Can you work these out from the model? Positions are in its coordinate system, mm. A direction names the side the tool comes from. Round coordinates to 2 decimals unless told otherwise and drop trailing zeros. Loops run counter-clockwise (first coordinate to the right, second up) from the corner with the lowest first, then second, coordinate; pieces in that order, holes last. Notation, with made-up numbers: (47.5, -33.75) - (61.5, -33.75) arc R14 cw to (61.5, -20.75) - close; hole circle Ø5 at (-22.75, -29.75). An arc over 180 degrees is marked (long way). Answer as CSV lines item,"result".
Autodesk Inventor part; units mm, degrees
ref_plane "YZ Plane" through (0, 0, 0) normal (1, 0, 0) x (0, 1, 0)
ref_plane "XZ Plane" through (0, 0, 0) normal (0, 1, 0) x (-1, 0, 0)
ref_plane "XY Plane" through (0, 0, 0) normal (0, 0, 1) x (1, 0, 0)
sketch "Sketch1" plane through (0, 0, 0) normal (0, 0, 1) x (1, 0, 0)
  line L0 (4, 0) -> (76, 0)
  line L1 (80, 4) -> (80, 87.5)
  line L2 (76, 91.5) -> (4, 91.5)
  line L3 (0, 87.5) -> (0, 4)
  line L4 (0, 4) -> (4, 0)
  line L5 (76, 0) -> (80, 4)
  line L6 (80, 87.5) -> (76, 91.5)
  line L7 (4, 91.5) -> (0, 87.5)
  line L8 (16.5, 75) -> (63.5, 75)
  line L9 (64.5, 74) -> (64.5, 65)
  line L10 (63.5, 64) -> (16.5, 64)
  line L11 (15.5, 65) -> (15.5, 74)
  arc A0 (15.5, 65) -> (16.5, 64) centre (16.5, 65) ccw
  arc A1 (16.5, 75) -> (15.5, 74) centre (16.5, 74) ccw
  arc A2 (64.5, 74) -> (63.5, 75) centre (63.5, 74) ccw
  arc A3 (63.5, 64) -> (64.5, 65) centre (63.5, 65) ccw
  line L12 (28.5, 21) -> (51.5, 21)
  line L13 (52.5, 20) -> (52.5, 11)
  line L14 (51.5, 10) -> (28.5, 10)
  line L15 (27.5, 11) -> (27.5, 20)
  arc A4 (27.5, 11) -> (28.5, 10) centre (28.5, 11) ccw
  arc A5 (28.5, 21) -> (27.5, 20) centre (28.5, 20) ccw
  arc A6 (52.5, 20) -> (51.5, 21) centre (51.5, 20) ccw
  arc A7 (51.5, 10) -> (52.5, 11) centre (51.5, 11) ccw
  line L16 (15.5, 69.5) -> (64.5, 69.5) construction
  line L17 (27.5, 15.5) -> (52.5, 15.5) construction
  circle A8 centre (40, 5) radius 2.25
  circle A9 centre (10, 78.5) radius 2.25
  circle A10 centre (6, 23.25) radius 2.25
  circle A11 centre (74, 23.25) radius 2.25
  circle A12 centre (70, 78.5) radius 2.25
  point P0 (0, 0)
  point P1 (40, 64)
  point P2 (40, 21)
  point P3 (40, 75)
  point P4 (40, 91.5)
  point P5 (0, 45.75)
  point P6 (80, 45.75)
  dimension "d0" = 45
  dimension "d1" = 4
  dimension "d2" = 1
  dimension "d3" = 11
  dimension "d4" = 49
  dimension "d5" = 1
  dimension "d6" = 11
  dimension "d7" = 25
  dimension "d9" = 10
  dimension "d10" = 16.5
  dimension "d11" = 4.5
  dimension "d12" = 4.5
  dimension "d13" = 5
  dimension "d15" = 4.5
  dimension "d16" = 4.5
  dimension "d19" = 54
  dimension "d22" = 80
  dimension "d23" = 6
  dimension "d24" = 6
  dimension "d25" = 23.25
  dimension "d26" = 4.5
  dimension "d27" = 10
  dimension "d28" = 10
  dimension "d54" = 3.5
extrude "Extrusion2" add sketch "Sketch1" along normal blind 6
sketch "Sketch2" plane through (0, 0, 6) normal (0, 0, 1) x (1, 0, 0)
  line L0 (4, 0) -> (76, 0)
  circle A0 centre (20, 35) radius 2.25
  circle A1 centre (60, 35) radius 2.25
  line L1 (20, 35) -> (60, 35) construction
  point P0 (0, 0)
  point P1 (40, 35)
  point P2 (40, 0)
  dimension "d31" = 4.5
  dimension "d32" = 4.5
  dimension "d33" = 40
  dimension "d34" = 35
extrude "Extrusion3" cut sketch "Sketch2" against normal through all
sketch "Sketch3" plane through (0, 0, 6) normal (0, 0, 1) x (1, 0, 0)
  circle A0 centre (20, 35) radius 2.25
  circle A1 centre (60, 35) radius 2.25
  line L0 (80, 4) -> (80, 87.5)
  line L1 (0, 87.5) -> (0, 4)
  line L2 (27.5, 38) -> (35.5, 38)
  line L3 (35.5, 38) -> (35.5, 32)
  line L4 (35.5, 32) -> (27.5, 32)
  line L5 (27.5, 32) -> (27.5, 38)
  line L6 (44.5, 38) -> (52.5, 38)
  line L7 (52.5, 38) -> (52.5, 32)
  line L8 (52.5, 32) -> (44.5, 32)
  line L9 (44.5, 32) -> (44.5, 38)
  line L10 (67.5, 38) -> (75.5, 38)
  line L11 (75.5, 38) -> (75.5, 32)
  line L12 (75.5, 32) -> (67.5, 32)
  line L13 (67.5, 32) -> (67.5, 38)
  line L14 (4.5, 38) -> (12.5, 38)
  line L15 (12.5, 38) -> (12.5, 32)
  line L16 (12.5, 32) -> (4.5, 32)
  line L17 (4.5, 32) -> (4.5, 38)
  line L18 (3, 16) -> (9, 16)
  line L19 (9, 16) -> (9, 8)
  line L20 (9, 8) -> (3, 8)
  line L21 (3, 8) -> (3, 16)
  line L22 (71, 16) -> (77, 16)
  line L23 (77, 16) -> (77, 8)
  line L24 (77, 8) -> (71, 8)
  line L25 (71, 8) -> (71, 16)
  point P0 (0, 0)
  point P1 (12.5, 35)
  dimension "d37" = 6
  dimension "d38" = 8
  dimension "d39" = 8
  dimension "d40" = 8
  dimension "d41" = 8
  dimension "d42" = 6
  dimension "d43" = 8
  dimension "d44" = 6
  dimension "d45" = 3
  dimension "d46" = 3
  dimension "d47" = 4
  dimension "d48" = 15
  dimension "d49" = 15
  dimension "d50" = 7.5
  dimension "d51" = 7.5
extrude "Extrusion4" cut sketch "Sketch3" against normal through all contours L2 L3 L4 L5 | L6 L7 L8 L9 | L10 L11 L12 L13 | L14 L15 L16 L17 | L18 L19 L20 L21 | L22 L23 L24 L25
sketch "Sketch4" plane through (0, 0, 6) normal (0, 0, 1) x (1, 0, 0)
  line L0 (4, 91.5) -> (76, 91.5)
  line L1 (76, 91.5) -> (76, 151.5)
  line L2 (36, 183.5) -> (4, 183.5)
  line L3 (4, 183.5) -> (4, 91.5)
  line L4 (36, 183.5) -> (36, 151.5)
  line L5 (36, 151.5) -> (76, 151.5)
  point P0 (0, 0)
  dimension "d55" = 92
  dimension "d57" = 32
  dimension "d58" = 32
extrude "Extrusion5" add sketch "Sketch4" against normal blind 6
chamfer "Chamfer1" distance 4 angle 45 1 edges at (76, 151.5, 3)
chamfer "Chamfer2" distance 2 angle 45 3 edges at (36, 151.5, 3) (36, 183.5, 3) (4, 183.5, 3)
sketch "Sketch5" plane through (0, 0, 6) normal (0, 0, 1) x (1, 0, 0)
  line L0 (4, 181.5) -> (4, 91.5)
  line L1 (34, 183.5) -> (6, 183.5)
  line L2 (10, 177.5) -> (24, 177.5) construction
  line L3 (24, 177.5) -> (24, 167.5) construction
  line L4 (24, 167.5) -> (10, 167.5) construction
  line L5 (10, 167.5) -> (10, 177.5) construction
  line L6 (15, 178.5) -> (19, 178.5)
  line L7 (23, 174.5) -> (23, 170.5)
  line L8 (19, 166.5) -> (15, 166.5)
  line L9 (11, 170.5) -> (11, 174.5)
  line L10 (11, 170.5) -> (15, 166.5)
  line L11 (19, 166.5) -> (23, 170.5)
  line L12 (23, 174.5) -> (19, 178.5)
  line L13 (15, 178.5) -> (11, 174.5)
  circle A0 centre (10, 177.5) radius 1.6
  circle A1 centre (10, 167.5) radius 1.6
  circle A2 centre (24, 167.5) radius 1.6
  circle A3 centre (24, 177.5) radius 1.6
  point P0 (0, 0)
  point P1 (23, 172.5)
  point P2 (24, 172.5)
  dimension "d67" = 45
  dimension "d68" = 4
  dimension "d69" = 3.2
  dimension "d70" = 14
  dimension "d71" = 10
  dimension "d72" = 1
  dimension "d73" = 1
  dimension "d74" = 6
  dimension "d75" = 6
extrude "Extrusion6" cut sketch "Sketch5" against normal through all
sketch "Sketch6" plane through (0, 0, 6) normal (0, 0, 1) x (1, 0, 0)
  line L0 (72, 151.5) -> (38, 151.5)
  line L1 (16.5, 75) -> (63.5, 75)
  line L2 (24.5, 148.5) -> (32.5, 148.5)
  line L3 (32.5, 148.5) -> (32.5, 142.5)
  line L4 (32.5, 142.5) -> (24.5, 142.5)
  line L5 (24.5, 142.5) -> (24.5, 148.5)
  line L6 (47.5, 148.5) -> (55.5, 148.5)
  line L7 (55.5, 148.5) -> (55.5, 142.5)
  line L8 (55.5, 142.5) -> (47.5, 142.5)
  line L9 (47.5, 142.5) -> (47.5, 148.5)
  line L10 (32.5, 148.5) -> (47.5, 142.5) construction
  line L11 (47.5, 148.5) -> (32.5, 142.5) construction
  circle A0 centre (40, 145.5) radius 2.25
  point P0 (0, 0)
  point P1 (40, 75)
  dimension "d78" = 6
  dimension "d79" = 8
  dimension "d80" = 8
  dimension "d81" = 15
  dimension "d82" = 4.5
  dimension "d83" = 3
extrude "Extrusion7" cut sketch "Sketch6" against normal through all
sketch "Sketch7" plane through (0, 0, 6) normal (0, 0, 1) x (1, 0, 0)
  line L0 (32.5, 142.5) -> (24.5, 142.5)
  line L1 (4, 181.5) -> (4, 91.5)
  line L2 (76, 91.5) -> (76, 147.5)
  line L3 (18, 139.5) -> (62, 139.5)
  line L4 (66, 135.5) -> (66, 95.5)
  line L5 (62, 91.5) -> (18, 91.5)
  line L6 (14, 95.5) -> (14, 135.5)
  line L7 (14, 135.5) -> (18, 139.5)
  line L8 (14, 95.5) -> (18, 91.5)
  line L9 (62, 91.5) -> (66, 95.5)
  line L10 (66, 135.5) -> (62, 139.5)
  point P0 (0, 0)
  point P1 (14, 139.5)
  point P2 (66, 91.5)
  point P3 (66, 139.5)
  point P4 (14, 91.5)
  dimension "d86" = 4
  dimension "d87" = 4
  dimension "d88" = 4
  dimension "d89" = 4
  dimension "d90" = 4
  dimension "d91" = 4
  dimension "d92" = 4
  dimension "d93" = 4
  dimension "d94" = 10
  dimension "d95" = 10
  dimension "d96" = 3
extrude "Extrusion8" cut sketch "Sketch7" against normal through all
equation "\"d95\" = d94"
properties part number "x_carriage_front"
Q1. On a 3-axis mill with a long thin cutter (end or side, diameter ignored), from which of +Z, -Z, +X, -X, +Y, -Y can I reach the whole of each face in a straight line? I mean faces 5 (the flat face through (15.5, 69, 3)), 6 (the flat face through (36, 168, 3)). Say none if no direction works.
Checks:
face 5,"+Z, -Z"
face 6,"+Z, -Z, +X, +Y"
Q2. I'm going to push flat-ended pins straight in: pin 1 Ø1 at (y, z) = (112, 1.5) entering from +X; pin 2 Ø3 at (x, z) = (47.5, 4) entering from +Y; pin 3 Ø3 at (y, z) = (173, 3) entering from +X. Where does each tip first touch, or does it pass through?
Checks:
pin 1,"x = 76"
pin 2,"y = 151.5"
pin 3,"x = 36"
Q3. Imagine slicing it at D-D (z = 3.7). Count the separate pieces of the cut face and the enclosed holes in it, then the cut area to 3 significant figures.
Checks:
separate pieces,"1"
enclosed holes,"24"
area,"8,690 mm²"
Q4. Imagine slicing it at A-A (y = 114). Write out the boundary of the cut face in (x, z), then the cut area to 3 significant figures.
Checks:
outline,"(4, 0) - (14, 0) - (14, 6) - (4, 6) - close; (66, 0) - (76, 0) - (76, 6) - (66, 6) - close"
area,"120 mm²"
Q5. Imagine slicing it at B-B (x = 40). Write out the boundary of the cut face in (y, z), then the cut area to 3 significant figures.
Checks:
outline,"(0, 0) - (2.75, 0) - (2.75, 6) - (0, 6) - close; (7.25, 0) - (10, 0) - (10, 6) - (7.25, 6) - close; (21, 0) - (64, 0) - (64, 6) - (21, 6) - close; (75, 0) - (91.5, 0) - (91.5, 6) - (75, 6) - close; (139.5, 0) - (143.25, 0) - (143.25, 6) - (139.5, 6) - close; (147.75, 0) - (151.5, 0) - (151.5, 6) - (147.75, 6) - close"
area,"435 mm²"
Q6. We'd pull the mould along Y, two halves only. Please class faces 1 (the flat face through (31, 38, 3)), 2 (the flat face through (71, 12, 3)), 3 (the flat face through (20, 183.5, 3)), 4 (the flat face through (39, 52, 0)): pulls with the +Y half, pulls with the -Y half, needs draft (parallel to the pull), parting line crosses it, or undercut.
Checks:
face 1,"undercut"
face 2,"undercut"
face 3,"pulls with the +Y half"
face 4,"needs draft"
Q7. If I drill on line 1 along Y through (x, z) = (40, 2.1); line 2 along X through (y, z) = (167.5, 2); line 3 along Y through (x, z) = (54, 0.8), over which ranges is the centre line in solid material (lowest first)? Write a range as [from, to].
Checks:
line 1,"[0, 2.75], [7.25, 10], [21, 64], [75, 91.5], [139.5, 143.25], [147.75, 151.5]"
line 2,"[4, 8.4], [11.6, 14], [20, 22.4], [25.6, 36]"
line 3,"[0, 64], [75, 91.5], [139.5, 142.5], [148.5, 151.5]"
Q8. Imagine slicing it at C-C (y = 23.25). Write out the boundary of the cut face in (x, z), then the cut area to 3 significant figures.
Checks:
outline,"(0, 0) - (3.75, 0) - (3.75, 6) - (0, 6) - close; (8.25, 0) - (71.75, 0) - (71.75, 6) - (8.25, 6) - close; (76.25, 0) - (80, 0) - (80, 6) - (76.25, 6) - close"
area,"426 mm²"
